```python
from build123d import *

# Parameters (mm, degrees)
SKETCH1_R           = 57
BOSS_EXTRUDE1_DEPTH = 3
SKETCH2_R           = 2
CUT_EXTRUDE1_DEPTH  = 81.665977958
CIRPATTERN1_COUNT   = 6
SKETCH5_R           = 3.25
BOSS_EXTRUDE2_DEPTH = 5
SKETCH4_R           = 16.5
CUT_EXTRUDE3_DEPTH  = 81.765091469
SKETCH8_R           = 2
CUT_EXTRUDE4_DEPTH  = 82.006172604
SKETCH9_R           = 3
CUT_EXTRUDE5_DEPTH  = 2.5
CUT_EXTRUDE7_DEPTH  = 2
CIRPATTERN3_COUNT   = 6
SKETCH12_R          = 25
SKETCH12_R_2        = 22.5
BOSS_EXTRUDE3_DEPTH = 2


with BuildPart() as part:
    # Sketch1 → Boss-Extrude1 (new body)
    with BuildSketch(Plane(origin=(0, 0, 0), x_dir=(1, 0, 0), z_dir=(0, 1, 0))):
        with Locations(Location((0, 0, 0), (0, 0, 270))):
            Circle(SKETCH1_R)
    extrude(amount=BOSS_EXTRUDE1_DEPTH)

    # Sketch2 → Cut-Extrude1 (cut, through all)
    with BuildSketch(Plane(origin=(0, 3, 0), x_dir=(1, 0, 0), z_dir=(0, 1, 0))):
        with Locations(Location((0, 46.5, 0), (0, 0, 270))):
            Circle(SKETCH2_R)
    cut_extrude1 = extrude(amount=-CUT_EXTRUDE1_DEPTH, mode=Mode.SUBTRACT)

    # CirPattern1: Cut-Extrude1 ×6 about axis
    cirpattern1_axis = Axis((0, 0, 0), (0, 1, 0))
    for i in range(1, CIRPATTERN1_COUNT):
        add(cut_extrude1.rotate(cirpattern1_axis, i * 360 / CIRPATTERN1_COUNT), mode=Mode.SUBTRACT)

    # Sketch5 → Boss-Extrude2 (add)
    with BuildSketch(Plane.XZ):
        with Locations(Location((0, 46.5, 0), (0, 0, 90))):
            Circle(SKETCH5_R)
        with Locations(Location((40.270181276, 23.25, 0), (0, 0, 90))):
            Circle(SKETCH5_R)
        with Locations(Location((40.270181276, -23.25, 0), (0, 0, 90))):
            Circle(SKETCH5_R)
        with Locations(Location((0, -46.5, 0), (0, 0, 90))):
            Circle(SKETCH5_R)
        with Locations(Location((-40.270181276, -23.25, 0), (0, 0, 90))):
            Circle(SKETCH5_R)
        with Locations(Location((-40.270181276, 23.25, 0), (0, 0, 90))):
            Circle(SKETCH5_R)
    extrude(amount=BOSS_EXTRUDE2_DEPTH)

    # Sketch4 → Cut-Extrude3 (cut, through all)
    with BuildSketch(Plane.XZ):
        with Locations(Location((0, 0, 0), (0, 0, 270))):
            Circle(SKETCH4_R)
    extrude(amount=-CUT_EXTRUDE3_DEPTH, mode=Mode.SUBTRACT)

    # Sketch8 → Cut-Extrude4 (cut, through all)
    with BuildSketch(Plane(origin=(0, 3, 0), x_dir=(1, 0, 0), z_dir=(0, 1, 0))):
        with Locations(Location((-40.270181276, -23.25, 0), (0, 0, 270))):
            Circle(SKETCH8_R)
        with Locations(Location((0, -46.5, 0), (0, 0, 270))):
            Circle(SKETCH8_R)
        with Locations(Location((40.270181276, -23.25, 0), (0, 0, 270))):
            Circle(SKETCH8_R)
        with Locations(Location((40.270181276, 23.25, 0), (0, 0, 270))):
            Circle(SKETCH8_R)
        with Locations(Location((0, 46.5, 0), (0, 0, 270))):
            Circle(SKETCH8_R)
        with Locations(Location((-40.270181276, 23.25, 0), (0, 0, 270))):
            Circle(SKETCH8_R)
    extrude(amount=-CUT_EXTRUDE4_DEPTH, mode=Mode.SUBTRACT)

    # Sketch9 → Cut-Extrude5 (cut)
    with BuildSketch(Plane(origin=(0, 3, 0), x_dir=(1, 0, 0), z_dir=(0, 1, 0))):
        with Locations(Location((-40.270181276, 23.25, 0), (0, 0, 270))):
            Circle(SKETCH9_R)
        with Locations(Location((0, 46.5, 0), (0, 0, 270))):
            Circle(SKETCH9_R)
        with Locations(Location((40.270181276, 23.25, 0), (0, 0, 270))):
            Circle(SKETCH9_R)
        with Locations(Location((40.270181276, -23.25, 0), (0, 0, 270))):
            Circle(SKETCH9_R)
        with Locations(Location((0, -46.5, 0), (0, 0, 270))):
            Circle(SKETCH9_R)
        with Locations(Location((-40.270181276, -23.25, 0), (0, 0, 270))):
            Circle(SKETCH9_R)
    extrude(amount=-CUT_EXTRUDE5_DEPTH, mode=Mode.SUBTRACT)

    # Sketch11 → Cut-Extrude7 (cut)
    with BuildSketch(Plane.XZ):
        with BuildLine():
            ThreePointArc((-50.023085711, 17.512592496), (-53, 0), (-50.023085711, -17.512592496))
            ThreePointArc((-50.023085711, -17.512592496), (-47.298125213, -20.050515589), (-43.662860234, -19.243476633))
            ThreePointArc((-43.662860234, -19.243476633), (-35.723547906, -20.625), (-38.496769739, -28.191407848))
            ThreePointArc((-38.496769739, -28.191407848), (-41.013318465, -30.936120192), (-40.177892843, -34.564966754))
            ThreePointArc((-40.177892843, -34.564966754), (-26.5, -45.899346401), (-9.845192868, -52.07755925))
            ThreePointArc((-9.845192868, -52.07755925), (-6.284806748, -50.98663578), (-5.166090495, -47.434884481))
            ThreePointArc((-5.166090495, -47.434884481), (0, -41.25), (5.166090495, -47.434884481))
            ThreePointArc((5.166090495, -47.434884481), (6.284806748, -50.98663578), (9.845192868, -52.07755925))
            ThreePointArc((9.845192868, -52.07755925), (26.5, -45.899346401), (40.177892843, -34.564966754))
            ThreePointArc((40.177892843, -34.564966754), (41.013318465, -30.936120192), (38.496769739, -28.191407848))
            ThreePointArc((38.496769739, -28.191407848), (35.723547906, -20.625), (43.662860234, -19.243476633))
            ThreePointArc((43.662860234, -19.243476633), (47.298125213, -20.050515589), (50.023085711, -17.512592496))
            ThreePointArc((50.023085711, -17.512592496), (53, 0), (50.023085711, 17.512592496))
            ThreePointArc((50.023085711, 17.512592496), (47.298125213, 20.050515589), (43.662860234, 19.243476633))
            ThreePointArc((43.662860234, 19.243476633), (35.723547906, 20.625), (38.496769739, 28.191407848))
            ThreePointArc((38.496769739, 28.191407848), (41.013318465, 30.936120192), (40.177892843, 34.564966754))
            ThreePointArc((40.177892843, 34.564966754), (26.5, 45.899346401), (9.845192868, 52.07755925))
            ThreePointArc((9.845192868, 52.07755925), (6.284806748, 50.98663578), (5.166090495, 47.434884481))
            ThreePointArc((5.166090495, 47.434884481), (0, 41.25), (-5.166090495, 47.434884481))
            ThreePointArc((-5.166090495, 47.434884481), (-6.284806748, 50.98663578), (-9.845192868, 52.07755925))
            ThreePointArc((-9.845192868, 52.07755925), (-26.5, 45.899346401), (-40.177892843, 34.564966754))
            ThreePointArc((-40.177892843, 34.564966754), (-41.013318465, 30.936120192), (-38.496769739, 28.191407848))
            ThreePointArc((-38.496769739, 28.191407848), (-35.723547906, 20.625), (-43.662860234, 19.243476633))
            ThreePointArc((-43.662860234, 19.243476633), (-47.298125213, 20.050515589), (-50.023085711, 17.512592496))
        make_face()
    cut_extrude7 = extrude(amount=-CUT_EXTRUDE7_DEPTH, mode=Mode.SUBTRACT)

    # CirPattern3: Cut-Extrude7 ×6 about axis
    cirpattern3_axis = Axis((0, 0, 0), (0, -1, 0))
    for i in range(1, CIRPATTERN3_COUNT):
        add(cut_extrude7.rotate(cirpattern3_axis, i * 360 / CIRPATTERN3_COUNT), mode=Mode.SUBTRACT)

    # Sketch12 → Boss-Extrude3 (add)
    with BuildSketch(Plane.XZ.offset(-2)):
        with Locations(Location((0, 0, 0), (0, 0, 270))):
            Circle(SKETCH12_R)
        with Locations(Location((0, 0, 0), (0, 0, 270))):
            Circle(SKETCH12_R_2, mode=Mode.SUBTRACT)
    extrude(amount=BOSS_EXTRUDE3_DEPTH)


solid = part.part
```
Input: part model. Units: mm. Frame: model coordinates. A direction names the side the tool comes from. Give positions to 0.01 mm unless a question says otherwise; leave off trailing zeros. Order: outer loops, then holes, each group sorted by start corner. A loop starts at its lowest first (then second) coordinate and runs counter-clockwise, first axis right, second up. Notation, with made-up numbers: M 38,31.5 L 84,31.5 A37 cw 84,68.5 Z; hole C 63.5,83.25 d2. An arc over 180 degrees is marked long. One line per question, with ' | ' between items. Start each with the question number.
1. Access query for faces 1 (the face through (-42, -5, 25)), 2 (the face through (-35.8, 1, -20.5)), 3 (the face through (0.1, 1.8, 43.5)). Directions: +Z, -Z, +X, -X, +Y, -Y. A direction counts if a zero-diameter tool reaches every point of the face in a straight line with its end or side. Return the directions, or none.
2. Section query D-D (x = 21). Return the cut outline in (y, z).
3. Section query C-C (x = 8.5). Return the cut outline in (y, z), and give its area (3 significant figures).
4. Pull-direction query (Z, two-part tool) for faces 4 (the face through (-12, 3, 12)), 5 (the face through (41.027, 0.986, -30.989)); classes: released by +Z, released by -Z, zero draft, split by the parting line, or undercut.
5. Section query B-B (z = 0). Return the cut outline in (x, y).
6. Material intervals for probe 1 along X at (y, z) = (-2.3, -23.25); probe 2 along X at (y, z) = (1.5, 0.5) (3 decimals); probe 3 along Z at (x, y) = (37.5, 0.75), sorted ascending. Write a range as [from, to].
7. First-contact query: pin 1 Ø3.5 at (x, z) = (-40.27, 23.25) entering from +Y; pin 2 Ø4 at (x, y) = (-13.5, 1.5) entering from +Z; pin 3 Ø5 at (x, z) = (0, 46.5) entering from +Y; pin 4 Ø4 at (y, z) = (2, 28) entering from +X. Flat tips, straight axial feed; report the tip coordinate or a pass-through.
8. Section query A-A (y = -2.25). Count the separate pieces of the cut face and the enclosed holes in it, and give its area (3 significant figures).
Here are the results:
1) face 1: +Z, -Z, +X, -X, -Y | face 2: -Y | face 3: +Y
2) outline: M 0,-52.99 L 3,-52.99 L 3,52.99 L 0,52.99 L 0,48.66 L 2,48.66 L 2,13.56 L 0,13.56 L 0,8.08 L 2,8.08 L 2,-8.08 L 0,-8.08 L 0,-13.56 L 2,-13.56 L 2,-48.66 L 0,-48.66 Z
3) outline: M 0,-56.36 L 3,-56.36 L 3,-14.14 L 2,-14.14 L 2,-20.83 L 0,-20.83 L 0,-23.51 L 2,-23.51 L 2,-52.1 L 0,-52.1 Z; M 0,20.83 L 2,20.83 L 2,14.14 L 3,14.14 L 3,56.36 L 0,56.36 L 0,52.1 L 2,52.1 L 2,23.51 L 0,23.51 Z | area: 112 mm²
4) face 4: zero draft | face 5: undercut
5) outline: M -57,0 L -53,0 L -53,2 L -25,2 L -25,0 L -22.5,0 L -22.5,2 L -16.5,2 L -16.5,3 L -57,3 Z; M 16.5,2 L 22.5,2 L 22.5,0 L 25,0 L 25,2 L 53,2 L 53,0 L 57,0 L 57,3 L 16.5,3 Z
6) probe 1: [-43.52, -42.27], [-38.27, -37.02], [37.02, 38.27], [42.27, 43.52] | probe 2: [-56.998, -52.998], [-24.995, -22.494], [22.494, 24.995], [52.998, 56.998] | probe 3: [-42.93, -37.45], [-27.71, -24.4], [-22.1, -18.79], [18.79, 22.1], [24.4, 27.71], [37.45, 42.93]
7) pin 1: through | pin 2: z = 55.83 | pin 3: y = 0.5 | pin 4: x = 50.72
8) separate pieces: 6 | enclosed holes: 6 | area: 124 mm²
